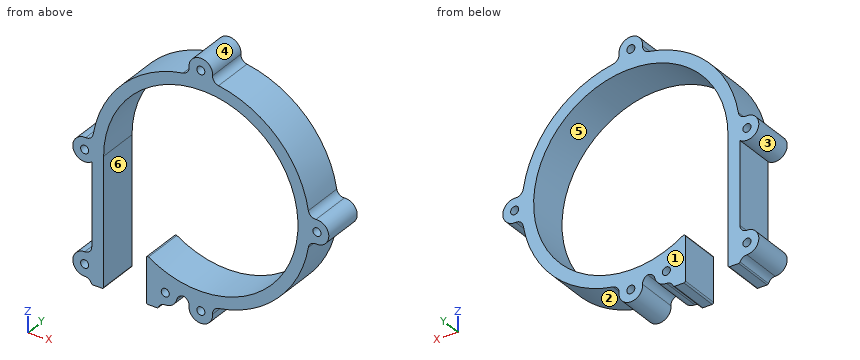
from build123d import *

# Parameters (mm, degrees)
SKETCH_1_R      = 1.7
EXTRUDE_1_DEPTH = 17.5
FILLET_1_R      = 3
FILLET_2_R      = 0.6


with BuildPart() as part:
    # 草图1 → 凸台-拉伸1 (new body)
    with BuildSketch(Plane(origin=(0, 0, 0), x_dir=(1, 0, 0), z_dir=(0, 1, 0))):
        with BuildLine():
            Line((-41, 0), (-41, 54))
            Line((-41, 54), (-46, 54))
            Line((-46, 54), (-46, 50.647615159))
            ThreePointArc((-46, 50.647615159), (-54, 46.647615159), (-46, 42.647615159))
            Line((-46, 42.647615159), (-46, 4))
            ThreePointArc((-46, 4), (-53.998925026, -0.103675394), (-45.836734694, -3.872176727))
            ThreePointArc((-45.836734694, -3.872176727), (-32.526911935, -32.526911935), (-3.872176727, -45.836734694))
            ThreePointArc((-3.872176727, -45.836734694), (0, -54), (3.872176727, -45.836734694))
            ThreePointArc((3.872176727, -45.836734694), (32.526911935, -32.526911935), (45.836734694, -3.872176727))
            ThreePointArc((45.836734694, -3.872176727), (54, 0), (45.836734694, 3.872176727))
            ThreePointArc((45.836734694, 3.872176727), (32.526911935, 32.526911935), (3.872176727, 45.836734694))
            ThreePointArc((3.872176727, 45.836734694), (0, 54), (-3.872176727, 45.836734694))
            ThreePointArc((-3.872176727, 45.836734694), (-7.126872346, 45.444556226), (-10.345371646, 44.821571654))
            ThreePointArc((-10.345371646, 44.821571654), (-11.971775359, 50.626290255), (-18, 50.647615159))
            Line((-18, 50.647615159), (-18, 54))
            Line((-18, 54), (-23, 54))
            Line((-23, 54), (-23, 33.941125497))
            ThreePointArc((-23, 33.941125497), (36.221540553, -19.209372712), (-41, 0))
        make_face()
        with Locations(Location((0, 49, 0), (0, 0, 270))):
            Circle(SKETCH_1_R, mode=Mode.SUBTRACT)
        with Locations(Location((49, 0, 0), (0, 0, 270))):
            Circle(SKETCH_1_R, mode=Mode.SUBTRACT)
        with Locations(Location((0, -49, 0), (0, 0, 270))):
            Circle(SKETCH_1_R, mode=Mode.SUBTRACT)
        with Locations(Location((-49, 0, 0), (0, 0, 270))):
            Circle(SKETCH_1_R, mode=Mode.SUBTRACT)
        with Locations(Location((-15, 46.647615159, 0), (0, 0, 270))):
            Circle(SKETCH_1_R, mode=Mode.SUBTRACT)
        with Locations(Location((-49, 46.647615159, 0), (0, 0, 270))):
            Circle(SKETCH_1_R, mode=Mode.SUBTRACT)
    extrude(amount=EXTRUDE_1_DEPTH)

    # 圆角1
    # the kernel refuses this fillet: 3 mm, written as the material it adds along each edge
    with BuildSketch(Plane(origin=(-3.872176727, 0, -45.836734694), x_dir=(-0.37402840247840613, 0, -0.9274172492138861), z_dir=(0, 1, 0)), Plane(origin=(45.836734694, 0, -3.872176727), x_dir=(0.9274172492138857, 0, -0.37402840247840763), z_dir=(0, 1, 0)), Plane(origin=(3.872176727, 0, 45.836734694), x_dir=(0.374028402478409, 0, 0.9274172492138849), z_dir=(0, 1, 0)), Plane(origin=(-45.836734694, 0, 3.872176727), x_dir=(-0.9274172492138864, 0, 0.3740284024784056), z_dir=(0, 1, 0))) as fillet_1_piece_1:
        with BuildLine():
            CenterArc((3.861943107, 2.864564734), FILLET_1_R, 167.400558819, 85.317583138)
            Line((0.934186439, 3.518965904), (0.875631305, 3.532053927))
            ThreePointArc((0.875631305, 3.532053927), (0.44393089, 1.765631899), (-0.057336629, 0.017677979))
            Line((-0.057336629, 0.017677979), (0.017824353, -0.057291295))
            ThreePointArc((0.017824353, -0.057291295), (1.485362734, 0.165725443), (2.952901114, -0.057291295))
            Line((2.952901114, -0.057291295), (2.970725467, 0))
        make_face()
    extrude(amount=17.5)
    with BuildSketch(Plane(origin=(3.872176727, 0, -45.836734694), x_dir=(0.9923388633046951, 0, 0.12354586344813656), z_dir=(0, 1, 0)), Plane(origin=(45.836734694, 0, 3.872176727), x_dir=(-0.12354586344813612, 0, 0.9923388633046951), z_dir=(0, 1, 0)), Plane(origin=(-3.872176727, 0, 45.836734694), x_dir=(-0.9923388633046952, 0, -0.12354586344813587), z_dir=(0, 1, 0)), Plane(origin=(-10.345371646, 0, -44.821571654), x_dir=(0.982518966413127, 0, -0.18616251136703332), z_dir=(0, 1, 0))) as fillet_1_piece_2:
        with BuildLine():
            CenterArc((3.759578561, 2.997649867), FILLET_1_R, 182.41437212, 85.317583138)
            Line((0.762241678, 2.871271047), (0.70229494, 2.868743471))
            ThreePointArc((0.70229494, 2.868743471), (0.541298099, 1.393112968), (-0.050799838, 0.031927676))
            Line((-0.050799838, 0.031927676), (0.002374471, -0.059952997))
            ThreePointArc((0.002374471, -0.059952997), (1.820427514, -0.023964621), (3.638480557, -0.059952997))
            Line((3.638480557, -0.059952997), (3.640855028, 0))
        make_face()
    extrude(amount=17.5)
    with BuildSketch(Plane(origin=(-46, 0, -42.647615159), x_dir=(-0.9486832980505127, 0, 0.31622776601684127), z_dir=(0, 1, 0))) as fillet_1_piece_3:
        with BuildLine():
            CenterArc((4.110960958, 2.846049894), FILLET_1_R, 161.565051177, 90)
            Line((1.264911064, 3.794733192), (1.207990066, 3.813706858))
            Line((1.207990066, 3.813706858), (-0.056920998, 0.018973666))
            Line((-0.056920998, 0.018973666), (0.018973666, -0.056920998))
            ThreePointArc((0.018973666, -0.056920998), (1.58113883, 0.19658351), (3.143303994, -0.056920998))
            Line((3.143303994, -0.056920998), (3.16227766, 0))
        make_face()
    extrude(amount=17.5)
    with BuildSketch(Plane(origin=(-46, 0, -50.647615159), x_dir=(1.5090941279718801e-12, 0, -1.0), z_dir=(0, 1, 0))) as fillet_1_piece_4:
        with BuildLine():
            CenterArc((3.99968789, 2.929334184), FILLET_1_R, 179.493886793, 78.04554374)
            Line((0.999804931, 2.955833865), (0.939807272, 2.956363859))
            ThreePointArc((0.939807272, 2.956363859), (0.679550236, 1.417151431), (-0.048, 0.036))
            Line((-0.048, 0.036), (0, -0.06))
            ThreePointArc((0, -0.06), (1.676192421, -0.06), (3.33943878, -0.058586684))
            Line((3.33943878, -0.058586684), (3.352384841, 0))
        make_face()
    extrude(amount=17.5)
    with BuildSketch(Plane(origin=(-18, 0, -50.647615159), x_dir=(0.9472773756522823, 0, -0.3204146900148692), z_dir=(0, 1, 0))) as fillet_1_piece_5:
        with BuildLine():
            CenterArc((4.056450754, 2.850212144), FILLET_1_R, 173.772564041, 78.04554374)
            Line((1.07415335, 3.175638315), (1.014507402, 3.182146838))
            ThreePointArc((1.014507402, 3.182146838), (0.480240032, 1.607044039), (-0.056836643, 0.019224881))
            Line((-0.056836643, 0.019224881), (0.01872208, -0.057004243))
            ThreePointArc((0.01872208, -0.057004243), (1.560173367, 0.189646427), (3.101624653, -0.057004243))
            Line((3.101624653, -0.057004243), (3.120346734, 0))
        make_face()
    extrude(amount=17.5)

    # 圆角2
    fillet_2_edges = [part.edges().sort_by_distance(p)[0] for p in [
        (-46, 8.75, -54),
        (-41, 8.75, -54),
        (-23, 8.75, -33.941125497),
        (-23, 8.75, -54),
        (-18, 8.75, -54),
    ]]
    fillet(fillet_2_edges, radius=FILLET_2_R)


solid = part.part
Input: part model. Units: mm. Frame: model coordinates. Face numbers are marked on the shaded views. A direction names the side the tool comes from. Coordinates: 2 decimals unless noted, no trailing zeros. Order: outer loops, then holes, each group sorted by start corner. A loop starts at its lowest first (then second) coordinate and runs counter-clockwise, first axis right, second up. Notation, with made-up numbers: M 52,33 L 60,33 A15 cw 60,62 Z; hole C 41,60 d5. An arc over 180 degrees is marked long. Answer as CSV lines item,"result".
1. Section D-D (y = 10.5). State how many separate pieces and enclosed holes the cut face has, then the cut area to 3 significant figures.
Reported:
separate pieces,"1"
enclosed holes,"6"
area,"1,850 mm2"
2. Pull-direction query (X, two-part tool) for the marked faces 1, 2, 3 and 4; classes: released by +X, released by -X, zero draft, split by the parting line, or undercut.
Reported:
face 1,"zero draft"
face 2,"released by +X"
face 3,"undercut"
face 4,"split by the parting line"
3. Section C-C (z = -33). Return the cut outline in (x, y).
Reported:
outline,"M -46,0 L -41,0 L -41,17.5 L -46,17.5 Z; M 24.33,0 L 32.05,0 L 32.05,17.5 L 24.33,17.5 Z"
4. Section A-A (x = 0). Return the cut outline in (y, z).
Reported:
outline,"M 0,-54 L 17.5,-54 L 17.5,-50.7 L 0,-50.7 Z; M 0,-47.3 L 17.5,-47.3 L 17.5,-41 L 0,-41 Z; M 0,41 L 17.5,41 L 17.5,47.3 L 0,47.3 Z; M 0,50.7 L 17.5,50.7 L 17.5,54 L 0,54 Z"
5. Access query for the marked faces 5 and 6. Directions: +Z, -Z, +X, -X, +Y, -Y. A direction counts if a zero-diameter tool reaches every point of the face in a straight line with its end or side. Return the directions, or none.
Reported:
face 5,"+Y, -Y"
face 6,"-Z, +Y, -Y"
6. First-contact query: P1, Ø10, axis at y = 7, z = -39.5, coming from the +X side; P2, Ø5, axis at y = 11, z = -18, coming from the -X side; P3, Ø1.5, axis at y = 7, z = -7.5, coming from the +X side. Flat tips, straight axial feed; report the tip coordinate or a pass-through.
Reported:
P1,"x = 30.43"
P2,"x = -46"
P3,"x = 45.61"
7. Material intervals for line 1 (X direction, y = 8.5, z = 49); line 2 (Z direction, x = 1, y = 15); line 3 (X direction, y = 13.75, z = -49), sorted ascending. Write a range as from..to.
Reported:
line 1,"-5..-1.7, 1.7..5"
line 2,"-53.9..-50.37, -47.63..-40.99, 40.99..47.63, 50.37..53.9"
line 3,"-53.41..-41, -23..-10.59, -5..-1.7, 1.7..5"
8. Section B-B (x = 12.5). Return the cut outline in (y, z).
Reported:
outline,"M 0,-44.27 L 17.5,-44.27 L 17.5,-39.05 L 0,-39.05 Z; M 0,39.05 L 17.5,39.05 L 17.5,44.27 L 0,44.27 Z"
